Verification items for the finished model (mm, model axes). Face numbers are marked on the shaded views. A direction names the side the tool comes from. Coordinates: 2 decimals unless noted, no trailing zeros. Order: outer loops, then holes, each group sorted by start corner. A loop starts at its lowest first (then second) coordinate and runs counter-clockwise, first axis right, second up. Notation, with made-up numbers: M 73.5,75.25 L 89.5,75.25 A28 ccw 89.5,95.25 Z; hole C -40,39 d8. An arc over 180 degrees is marked long. Return JSON: item names as keys, results as strings. Group by question number.
Q1. Section check D-D, the plane z = 89. Enter the section's corners in (x, y).
Q2. Thickness scan on probe 1 along Z at (x, y) = (-23, -18); probe 2 along Y at (x, z) = (-15, 93); probe 3 along Z at (x, y) = (-27.5, -16.5). Record the ranges inside material, lowest first.
Q3. Access from +Z, -Z, +X, -X, +Y, -Y to the whole of each face (thin tool, end or side, straight path). Record for the marked faces 5, 6 and 7.
Q4. Section check B-B, the plane x = -23. Enter the section's corners in (y, z), then the cut area to 3 significant figures.
Q5. Section check C-C, the plane z = 110. Enter the section's corners in (x, y).
Q6. Section check A-A, the plane y = -10. Enter the section's corners in (x, z).
Q7. Mould release check, pull along Z, two halves, no side actions. Record for the marked faces 1, 2, 3 and 4: pulls with the +Z half, pulls with the -Z half, needs draft (parallel to the pull), parting line crosses it, or undercut.
Q8. Go/stop test with flat-tipped pins: pin 1 Ø6 at (x, y) = (-25, -7) entering from +Z; pin 2 Ø18 at (x, z) = (-42.5, 68) entering from +Y; pin 3 Ø6 at (x, y) = (-25.5, 1.5) entering from -Z. Record where each tip stops, or that it passes through.
from build123d import *

# Parameters (mm, degrees)
F0_W     = 63
F0_H     = 150
F0_R     = 10
F0_W_2   = 20
F0_H_2   = 20
F1_DEPTH = 20
F2_T     = -3
F3_R     = 5
F4_DEPTH = 5
F5_SIZE  = 3


with BuildPart() as f1:
    # F0 (on Front) → F1 (new body)
    with BuildSketch(Plane.XZ):
        with Locations((-31.5, 75)):
            Rectangle(F0_W, F0_H)
        with Locations((-23, 30)):
            Circle(F0_R, mode=Mode.SUBTRACT)
        with Locations((-23, 110)):
            Rectangle(F0_W_2, F0_H_2, mode=Mode.SUBTRACT)
    extrude(amount=F1_DEPTH)

    # F2
    f2_openings = [f1.faces().sort_by_distance(p)[0] for p in [
        (-63, -10, 75),
        (-13, -10, 110),
        (-23, -10, 100),
        (-33, -10, 110),
        (-23, -10, 120),
        (-33, -10, 30),
    ]]
    offset(amount=F2_T, openings=f2_openings)

    # F3 (on face) → F4 (join)
    with BuildSketch(Plane(origin=(-63, 0, 0), x_dir=(0, -1, 0), z_dir=(-1, 0, 0))):
        with BuildLine():
            ThreePointArc((25, 163), (21.485281, 171.485281), (13, 175))
            Line((13, 175), (7, 175))
            ThreePointArc((7, 175), (-1.485281, 171.485281), (-5, 163))
            Line((-5, 163), (-5, -13))
            ThreePointArc((-5, -13), (-1.485281, -21.485281), (7, -25))
            Line((7, -25), (13, -25))
            ThreePointArc((13, -25), (21.485281, -21.485281), (25, -13))
            Line((25, -13), (25, 163))
        make_face()
        with Locations((10, -13)):
            Circle(F3_R, mode=Mode.SUBTRACT)
        with Locations((10, 163)):
            Circle(F3_R, mode=Mode.SUBTRACT)
    extrude(amount=F4_DEPTH)

    # F5
    f5_edges = [f1.edges().sort_by_distance(p)[0] for p in [
        (-68, -5, 163),
        (-68, -5, -13),
    ]]
    chamfer(f5_edges, length=F5_SIZE)


solid = f1.part
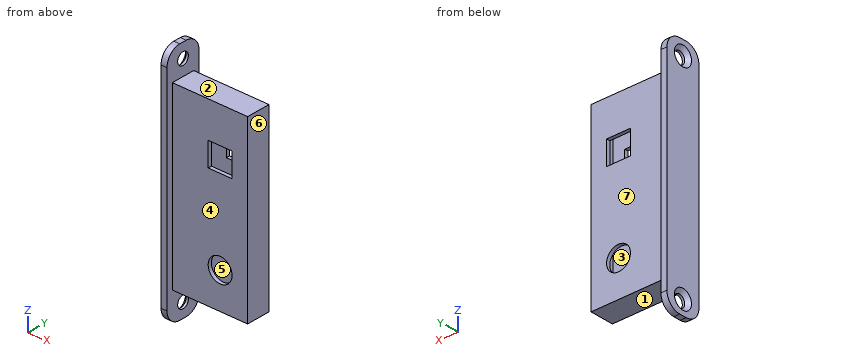
Numbers:
{
 "1": {"outline": "M -68,-25 L -63,-25 L -63,-20 L 0,-20 L 0,0 L -63,0 L -63,5 L -68,5 Z; hole M -63,-17 L -3,-17 L -3,-3 L -63,-3 Z"},
 "2": {"probe 1": "z = 0 to 20, 40 to 100, 120 to 150", "probe 2": "y = -20 to -17, -3 to 0", "probe 3": "z = 0 to 3, 147 to 150"},
 "3": {"face 5": "none", "face 6": "+Z, -Z, +X, +Y, -Y", "face 7": "+Z, -Z, +X, +Y"},
 "4": {"outline": "M -20,0 L 0,0 L 0,20 L -3,20 L -3,3 L -17,3 L -17,20 L -20,20 Z; M -20,40 L -17,40 L -17,100 L -20,100 Z; M -20,120 L -17,120 L -17,147 L -3,147 L -3,120 L 0,120 L 0,150 L -20,150 Z; M -3,40 L 0,40 L 0,100 L -3,100 Z", "area": "744 mm2"},
 "5": {"outline": "M -68,-25 L -63,-25 L -63,-20 L -33,-20 L -33,-17 L -63,-17 L -63,-3 L -33,-3 L -33,0 L -63,0 L -63,5 L -68,5 Z; M -13,-20 L 0,-20 L 0,0 L -13,0 L -13,-3 L -3,-3 L -3,-17 L -13,-17 Z"},
 "6": {"outline": "M -68,-25 L -63,-25 L -63,-18 L -65,-18 L -68,-21 Z; M -68,-5 L -65,-8 L -63,-8 L -63,0 L 0,0 L 0,150 L -63,150 L -63,158 L -65,158 L -68,155 Z; M -68,171 L -65,168 L -63,168 L -63,175 L -68,175 Z; hole M -63,3 L -3,3 L -3,147 L -63,147 Z"},
 "7": {"face 1": "pulls with the -Z half", "face 2": "pulls with the +Z half", "face 3": "undercut", "face 4": "needs draft"},
 "8": {"pin 1": "stops at z = 150", "pin 2": "stops at y = 0", "pin 3": "stops at z = 0"}
}
